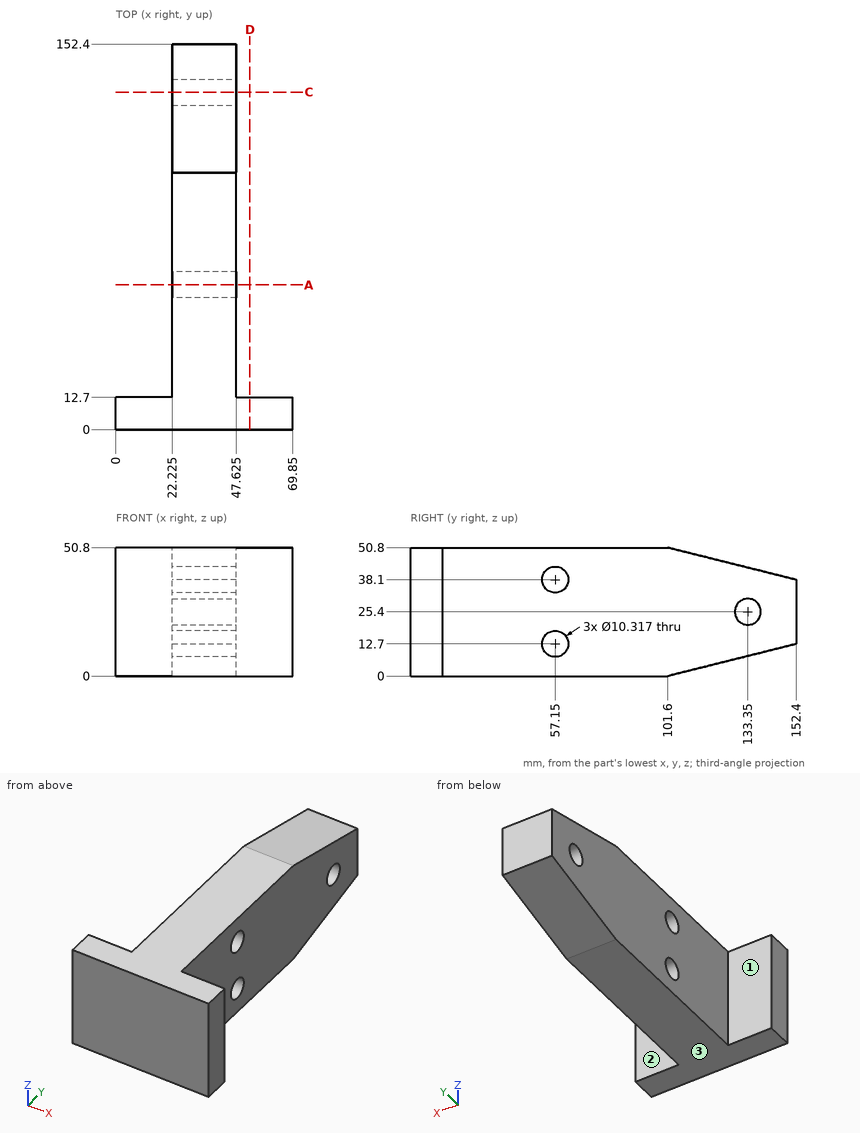
Study the drawing (mm; zero at the part's minimum x, y, z) and answer. A direction names the side the tool comes from. Coordinates: 2 decimals unless noted, no trailing zeros. Loops run counter-clockwise (first coordinate to the right, second up) from the corner with the lowest first, then second, coordinate; pieces in that order, holes last. Notation, with made-up numbers: (33.5, 57) -> (77.5, 57) arc R20 ccw to (77.5, 93) -> close; hole circle Ø3 at (-30, 3.5). An arc over 180 degrees is marked (long way). Write each question's results on one line, items separated by ' | '. Start each with the question number.
1) Find section A-A on y = 57.15. Determine the outline of the cut face in (x, z) (1 decimal), then the cut area to 3 significant figures.
2) Find section D-D on x = 53. Determine the outline of the cut face in (y, z).
3) For the marked faces 1, 2 and 3, determine the directions among +Z, -Z, +X, -X, +Y, -Y from which every point of the face is accessible in a straight line to the end or side of a thin tool.
4) Flat-ended cylindrical pins translate along their axes: P1, Ø4, axis at x = 21, z = 36, coming from the -Y side; P2, Ø12, axis at y = 57.15, z = 38.1, coming from the +X side (1 decimal); P3, Ø11, axis at x = 16, z = 14.5, coming from the +Y side; P4, Ø1, axis at y = 124.5, z = 37.5, coming from the -X side (1 decimal). Find the tip coordinate at first contact, or state that the pin passes through.
5) Find section C-C on y = 133.35. Determine the outline of the cut face in (x, z) (1 decimal).
6) Consider line 1 along Y through (x, z) = (36, 38); line 2 along Y through (x, z) = (33, 25.4); line 3 along Z through (x, y) = (36.5, 54) (1 decimal). Determine where each line is inside the solid, lowest interval first.
Response values:
1) outline: (22.2, 0) -> (47.6, 0) -> (47.6, 7.5) -> (22.2, 7.5) -> close; (22.2, 17.9) -> (47.6, 17.9) -> (47.6, 32.9) -> (22.2, 32.9) -> close; (22.2, 43.3) -> (47.6, 43.3) -> (47.6, 50.8) -> (22.2, 50.8) -> close | area: 766 mm^2
2) outline: (0, 0) -> (12.7, 0) -> (12.7, 50.8) -> (0, 50.8) -> close
3) face 1: +Z, -Z, -X, +Y | face 2: +Z, -Z, +X, +Y | face 3: -Z, +X, -X, +Y, -Y
4) P1: stops at y = 0 | P2: stops at x = 47.6 | P3: stops at y = 12.7 | P4: stops at x = 22.2
5) outline: (22.2, 7.9) -> (47.6, 7.9) -> (47.6, 20.2) -> (22.2, 20.2) -> close; (22.2, 30.6) -> (47.6, 30.6) -> (47.6, 42.9) -> (22.2, 42.9) -> close
6) line 1: y = 0 to 51.99, 62.31 to 152.4 | line 2: y = 0 to 128.19, 138.51 to 152.4 | line 3: z = 0 to 8.6, 16.8 to 34, 42.2 to 50.8
